Autodesk Fusion 360 part; units mm, degrees
sketch "Sketch1" plane through (0, 0, 0) normal (1, 0, 0) x (0, 1, 0)
  circle A0 centre (0, 0) radius 5
  dimension "d1" = 10
extrude "Extrude1" add sketch "Sketch1" along normal blind 180
sketch "Sketch2" plane through (180, 0, 0) normal (1, 0, 0) x (0, 1, 0)
  circle A0 centre (0, 0) radius 5
  circle A1 centre (0, 0) radius 4
  dimension "d4" = 8
extrude "Extrude2" cut sketch "Sketch2" against normal blind 20
sketch "Sketch3" plane through (0, 0, 0) normal (-1, 0, 0) x (0, -1, 0)
  circle A0 centre (0, 0) radius 5
  circle A1 centre (0, 0) radius 4
  dimension "d7" = 8
extrude "Extrude3" cut sketch "Sketch3" against normal blind 100
extrude "Extrude4" add 1 faces at (160, 4.6332, -0.4471) along direction (1, 0, 0) blind 5
extrude "Extrude5" cut 1 faces at (180, -1.2456, 0.0132) along direction (-1, 0, 0) blind 5
extrude "Extrude6" add 1 faces at (175, -1.2456, 0.0132) along direction (1, 0, 0) blind 26
extrude "Extrude7" add 1 faces at (165, 4.6332, -0.4471) along direction (1, 0, 0) blind 26
extrude "Extrude8" add 1 faces at (100, 4.6332, 0.4471) along direction (-1, 0, 0) blind 26
extrude "Extrude9" cut 1 faces at (0, 0.2111, 0.732) along direction (1, 0, 0) blind 30.1
extrude "Extrude10" add 1 faces at (30.1, 0.2111, 0.732) along direction (-1, 0, 0) blind 0.1
extrude "Extrude11" cut 1 faces at (30, 0.2111, 0.732) along direction (1, 0, 0) blind 1
extrude "Extrude12" add 1 faces at (31, 0.2111, 0.732) along direction (-1, 0, 0) blind 10
extrude "Extrude13" add 1 faces at (21, 0.2111, 0.732) along direction (-1, 0, 0) blind 10
sketch "Sketch4" plane through (0, 0, 0) normal (0, 0, 1) x (1, 0, 0)
  line L0 (191, 0) -> (186, 0)
  circle A0 centre (186, 0) radius 2.25
  circle A1 centre (161, 0) radius 2.25
  dimension "d30" = 5
  dimension "d31" = 4.5
  dimension "d35" = 4.5
sketch "Sketch5" plane through (0, 0, 0) normal (0, 0, 1) x (1, 0, 0)
  circle A0 centre (161, 0) radius 2.25
  line L0 (191, -5) -> (191, 5)
  dimension "d38" = 4.5
  dimension "d39" = 30
extrude "Extrude17" add 1 faces at (11, 0.2111, 0.732) along direction (-1, 0, 0) blind 63
extrude "Extrude18" add 1 faces at (74, 4.6332, 0.4471) along direction (-1, 0, 0) blind 63
extrude "Extrude19" add 1 faces at (-52, 0.2111, 0.732) along direction (-1, 0, 0) blind 37
extrude "Extrude20" cut 1 faces at (201, -1.2456, 0.0132) along direction (-1, 0, 0) blind 3
sketch "Sketch6" plane through (0, 0, 0) normal (0, 0, 1) x (1, 0, 0)
  line L0 (190, 0) -> (105, 0)
  circle A0 centre (105, 0) radius 2.25
  dimension "d50" = 4.5
extrude "Extrude21" cut sketch "Sketch6" along normal mid plane 20
Design review of the part built by this model. Coordinates are the model's own, in mm. A direction names the side the tool comes from. Round coordinates to 2 decimals unless told otherwise and drop trailing zeros. Write each loop counter-clockwise with the first axis right and the second up, starting at its lowest first coordinate (ties: lowest second). Pieces come first, ordered by that corner, then holes. Notation, with made-up numbers: (-18.5, -12) -> (5.5, -12) arc R35 cw to (5.5, 24) -> close; hole circle Ø11 at (83, 67). An arc over 180 degrees is marked (long way). Answer in a Markdown table with one row per item.
Q1. Take a section at A-A, the plane y = 0. State the section outline as (x, z) points, then the cut area to 3 significant figures.
The answers:
| item | result |
|---|---|
| outline | (-89, -4) -> (11, -4) -> (11, -5) -> (102.75, -5) -> (102.75, 5) -> (11, 5) -> (11, 4) -> (-89, 4) -> close; (107.25, -5) -> (191, -5) -> (191, -4) -> (198, -4) -> (198, 4) -> (191, 4) -> (191, 5) -> (107.25, 5) -> close |
| area | 2,610 mm² |
Q2. To check wall thickness, follow L1, parallel to X at y = 0, z = -2.5; L2, parallel to X at y = 0.25, z = 4.5; L3, parallel to Y at x = 12, z = 3. State the ranges of each line that lie inside material, in increasing order. Write a range as [from, to].
The answers:
| item | result |
|---|---|
| L1 | [-89, 102.75], [107.25, 198] |
| L2 | [11, 102.76], [107.24, 191] |
| L3 | [-4, 4] |
Q3. Draft analysis for pull direction X (two halves, no side actions). For faces 1 (the face through (-89, 0, 0)), 2 (the face through (107.08, 0.86, -0.07)), 3 (the face through (-38.3, 0.867, 3.905)), state which applies: +X half, -X half, draft (parallel to the pull), parting line (faces both ways), or undercut.
The answers:
| item | result |
|---|---|
| face 1 | -X half |
| face 2 | undercut |
| face 3 | draft |
Q4. Take a section at D-D, the plane x = -40. State the section outline as (y, z) points, then the cut area to 3 significant figures.
The answers:
| item | result |
|---|---|
| outline | circle Ø8 at (0, 0) |
| area | 50.3 mm² |
Q5. Take a section at C-C, the plane x = 74. State the section outline as (y, z) points.
The answers:
| item | result |
|---|---|
| outline | circle Ø10 at (0, 0) |
Q6. For faces 4 (the face through (194.451, -0.867, 3.905)), 5 (the face through (198, 0, 0)), list the 3-axis set-ups (+Z, -Z, +X, -X, +Y, -Y) from which the entire face can be reached by the end or side of a thin tool; tool diameter is ignored.
The answers:
| item | result |
|---|---|
| face 4 | +X |
| face 5 | +Z, -Z, +X, +Y, -Y |
Q7. Take a section at B-B, the plane z = 2.25. State the section outline as (x, y) points, then the cut area to 3 significant figures.
The answers:
| item | result |
|---|---|
| outline | (-89, -3.31) -> (11, -3.31) -> (11, -4.47) -> (191, -4.47) -> (191, -3.31) -> (198, -3.31) -> (198, 3.31) -> (191, 3.31) -> (191, 4.47) -> (11, 4.47) -> (11, 3.31) -> (-89, 3.31) -> close; hole circle Ø4.5 at (105, 0) |
| area | 2,300 mm² |
Q8. Clearance check with flat-ended pins moving along their axes: pin 1 Ø6 at (x, y) = (66.5, 2) entering from +Z; pin 2 Ø2 at (x, y) = (4.5, 0) entering from -Z. State where each tip first meets the part, or that it passes through.
The answers:
| item | result |
|---|---|
| pin 1 | z = 5 |
| pin 2 | z = -4 |
